from build123d import *

# Parameters (mm, degrees)
F0_R     = 1.5
F1_DEPTH = 6
F0_R_2   = 2.25
F2_DEPTH = 4.1
F0_R_3   = 6
F3_DEPTH = 4
F4_SIZE  = 1


# Not quite as in the source:
# - a fillet or chamfer that OpenCascade refuses, or shapes differently, is made with other operations: its cross-section is extruded or revolved along the edge and cut away or added


with BuildPart() as f1:
    # F0 (on Top) → F1 (new body)
    with BuildSketch(Plane.XY):
        Circle(F0_R)
    extrude(amount=F1_DEPTH)

    # F0 (on Top) → F2 (join)
    with BuildSketch(Plane.XY):
        Circle(F0_R_2)
        Circle(F0_R, mode=Mode.SUBTRACT)
    extrude(amount=F2_DEPTH)

    # F0 (on Top) → F3 (join)
    with BuildSketch(Plane.XY):
        Circle(F0_R_3)
        Circle(F0_R_2, mode=Mode.SUBTRACT)
    extrude(amount=F3_DEPTH)

    # F4
    f4_edges = [f1.edges().sort_by_distance(p)[0] for p in [
        (-6, 0, 4),
    ]]
    chamfer(f4_edges, length=F4_SIZE)

    # F5: chamfer of 2 on 1 edges, made by hand

    # F5_s1 → F5_t2 (revolve, cut)
    with BuildSketch(Plane.XZ):
        Polygon((3, 4), (6.4142135624, 2.5857864376), (5, 4), align=None)
    revolve(axis=Axis((0, 0, 4), (0, 0, 1)), mode=Mode.SUBTRACT)


solid = f1.part
CAD build for the part. Positions are in the model's coordinates, mm. A direction names the side the tool comes from. Round coordinates to 2 decimals unless told otherwise and drop trailing zeros. Loops run counter-clockwise (first coordinate to the right, second up) from the corner with the lowest first, then second, coordinate; pieces in that order, holes last.
(1) Cut at C-C (z = 2.3). Give the cut face in (x, y), plus the area to 3 significant figures.
(2) Which spindle directions (+Z, -Z, +X, -X, +Y, -Y) get a long thin tool onto all of the face, cutting with end or side? Do faces 1 (the flat face through (0, 0, 0)), 2 (the flat face through (-2, 0, 4.1)). Say none if no direction does.
(3) Cut at D-D (z = 3.5). Give the cut face in (x, y).
(4) Cut at A-A (y = 0). Give the cut face in (x, z).
(5) Drop flat-ended pins along their axis: pin 1 (2 mm diameter, centred on y = -3, z = 1, fed in from +X); pin 2 (1.5 mm diameter, centred on x = -1.5, z = 1, fed in from -Y); pin 3 (1 mm diameter, centred on x = -3, y = -2.5, fed in from +Z). Give the stop position or say it passes through.
(6) Wall check: line 1 along Z through (x, y) = (-0.75, -2.5); line 2 along Y through (x, z) = (-0.5, 4.6); line 3 along Z through (x, y) = (-5.5, 0.25). Give the ranges that are in metal, low to high.
Findings below:
1. outline: circle Ø12 at (0, 0)
1. area: 113 mm2
2. face 1: -Z, +X, -X, +Y, -Y
2. face 2: +Z
3. outline: circle Ø8.41 at (0, 0)
4. outline: (-6, 0) - (6, 0) - (6, 2.76) - (3, 4) - (2.25, 4) - (2.25, 4.1) - (1.5, 4.1) - (1.5, 6) - (-1.5, 6) - (-1.5, 4.1) - (-2.25, 4.1) - (-2.25, 4) - (-3, 4) - (-6, 2.76) - close
5. pin 1: stops at x = 5.66
5. pin 2: stops at y = -5.95
5. pin 3: stops at z = 3.83
6. line 1: z = 0 to 4
6. line 2: y = -1.41 to 1.41
6. line 3: z = 0 to 2.96
